Verification items for the finished model (mm, model axes). A direction names the side the tool comes from. Give positions to 0.01 mm unless a question says otherwise; leave off trailing zeros. Write each loop counter-clockwise with the first axis right and the second up, starting at its lowest first coordinate (ties: lowest second). Pieces come first, ordered by that corner, then holes. Notation, with made-up numbers: (47.25, 25.25) -> (106.25, 25.25) arc R17 ccw to (106.25, 37.25) -> close; hole circle Ø5 at (-32.5, 79.25). An arc over 180 degrees is marked (long way). Use one line per item in the form item = value. Start each with the question number.
(1) Section check C-C, the plane x = -25198.5. Record the cut outline in (y, z), plus the area to 3 significant figures.
(2) Set-up check for faces 1 (the face through (-25284.553, 8816, 1)), 2 (the face through (-25216, 8811, 0)), 3 (the face through (-25144.553, 8806, 1)): record each of +Z, -Z, +X, -X, +Y, -Y from which the full face is reachable in a straight line by a thin tool's end or side.
(3) Scan lines: L1, parallel to X at y = 8806, z = 1.5; L2, parallel to Z at x = -25220, y = 8807.25; L3, parallel to X at y = 8815, z = 1.5. Record each from-to range of solid material in increasing order.
(4) Depth check by flat-ended pin: pin 1 Ø8 at (x, y) = (-25213.5, 8808) entering from +Z; pin 2 Ø1.2 at (x, z) = (-25285.88, 1.5) entering from -Y; pin 3 Ø6 at (x, y) = (-25216, 8816) entering from -Z. Enter the tip coordinate at first touch or a pass-through.
(5) Section check A-A, the plane z = 1.5. Record the cut outline in (x, y).
(6) Section check B-B, the plane y = 8815.5. Record the cut outline in (x, z).
from build123d import *

# Parameters (mm, degrees)
SKETCH1_W           = 140
SKETCH1_H           = 20
BOSS_EXTRUDE1_DEPTH = 3
SKETCH2_R           = 2
SKETCH2_R_2         = 1
BOSS_EXTRUDE2_DEPTH = 10
SKETCH3_R           = 2
SKETCH3_R_2         = 1
BOSS_EXTRUDE3_DEPTH = 10


with BuildPart() as part:
    # Sketch1 → Boss-Extrude1 (new body)
    with BuildSketch(Plane.XY):
        with Locations((-25214.552845528, 8811.138211382)):
            Rectangle(SKETCH1_W, SKETCH1_H)
    extrude(amount=BOSS_EXTRUDE1_DEPTH)

    # Sketch2 → Boss-Extrude2 (add)
    with BuildSketch(Plane(origin=(0, 8821.138211382, 0), x_dir=(1, 0, 0), z_dir=(0, 1, 0))):
        with Locations((-25143.229969873, -1.5)):
            Circle(SKETCH2_R)
        with Locations(Location((-25143.229969873, -1.5, 0), (0, 0, 89.999999998))):
            Circle(SKETCH2_R_2, mode=Mode.SUBTRACT)
    extrude(amount=-BOSS_EXTRUDE2_DEPTH)

    # Sketch3 → Boss-Extrude3 (add)
    with BuildSketch(Plane.XZ.offset(-8801.138211382)):
        with Locations((-25285.875721184, 1.5)):
            Circle(SKETCH3_R)
        with Locations(Location((-25285.875721184, 1.5, 0), (0, 0, 270))):
            Circle(SKETCH3_R_2, mode=Mode.SUBTRACT)
    extrude(amount=-BOSS_EXTRUDE3_DEPTH)


solid = part.part
Completed:
q1.outline = (8801.14, 0) -> (8821.14, 0) -> (8821.14, 3) -> (8801.14, 3) -> close
q1.area = 60.0 mm²
q2.face_1 = +Z, -Z, -X, +Y
q2.face_2 = -Z, +Y, -Y
q2.face_3 = +Z, -Z, +X, -Y
q3.L1 = -25287.88 to -25286.88, -25284.88 to -25144.55
q3.L2 = 0 to 3
q3.L3 = -25284.55 to -25144.23, -25142.23 to -25141.23
q4.pin_1 = 3
q4.pin_2 = through
q4.pin_3 = 0
q5.outline = (-25287.88, 8801.14) -> (-25286.88, 8801.14) -> (-25286.88, 8811.14) -> (-25287.88, 8811.14) -> close; (-25284.88, 8801.14) -> (-25144.55, 8801.14) -> (-25144.55, 8811.14) -> (-25144.23, 8811.14) -> (-25144.23, 8821.14) -> (-25284.55, 8821.14) -> (-25284.55, 8811.14) -> (-25284.88, 8811.14) -> close; (-25142.23, 8811.14) -> (-25141.23, 8811.14) -> (-25141.23, 8821.14) -> (-25142.23, 8821.14) -> close
q6.outline = (-25284.55, 0) -> (-25144.55, 0) arc R2 ccw (long way) to (-25144.55, 3) -> (-25284.55, 3) -> close; hole circle Ø2 at (-25143.23, 1.5)
